CAD build for the part. Positions are in the model's coordinates, mm. A direction names the side the tool comes from. Give positions to 0.01 mm unless a question says otherwise; leave off trailing zeros. Loops run counter-clockwise (first coordinate to the right, second up) from the corner with the lowest first, then second, coordinate; pieces in that order, holes last. Notation, with made-up numbers: (-36, -1.5) -> (-29, -1.5) arc R9 cw to (-29, 7.5) -> close; hole circle Ø8 at (39, 70.25). An arc over 180 degrees is marked (long way). Write each question's results on one line, items separated by ' | '. Start each with the question number.
```python
from build123d import *

# Parameters (mm, degrees)
SKETCH_1_R          = 42
EXTRUDE_1_DEPTH     = 20
EXTRUDE_2_DEPTH     = 5
SKETCH_4_R          = 42
CUT_EXTRUDE_1_DEPTH = 15
SKETCH_5_R          = 42
EXTRUDE_3_DEPTH     = 10


with BuildPart() as part:
    # Sketch 1 → Extrude 1 (new body)
    with BuildSketch(Plane.XY):
        Circle(SKETCH_1_R)
    extrude(amount=EXTRUDE_1_DEPTH)



with BuildPart() as body_2:
    # Sketch 2 → Revolve 1 (revolve)
    with BuildSketch(Plane.XY.offset(20), mode=Mode.PRIVATE) as revolve_1_sk:
        with BuildLine():
            Line((100, 20), (100, 15))
            ThreePointArc((100, 15), (86.583592135, 6.708203932), (88, -9))
            Line((88, -9), (80, -9))
            Line((80, -9), (80, 20))
            Line((80, 20), (100, 20))
        make_face()
    revolve(revolve_1_sk.sketch.rotate(Axis((100, 22.717290725, 20), (0, -1, 0)), 270), axis=Axis((100, 22.717290725, 20), (0, -1, 0)))


with BuildPart() as part_1:
    add(part.part)

    add(body_2.part)  # Extrude 2 merges body 2
    # Sketch 3 → Extrude 2 (add, symmetric)
    with BuildSketch(Plane.XY.offset(20)):
        with BuildLine():
            Line((14.069453744, 39.573355574), (86, 14))
            Line((86, 14), (86, -3))
            Line((86, -3), (19.208719722, -37.350034627))
            ThreePointArc((19.208719722, -37.350034627), (-41.906577017, -2.79978619), (14.069453744, 39.573355574))
        make_face()
    extrude(amount=EXTRUDE_2_DEPTH, both=True)

    # Sketch 4 → Cut-Extrude 1 (cut)
    with BuildSketch(Plane(origin=(0, 0, 0), x_dir=(-1, 0, 0), z_dir=(0, 0, -1))):
        Circle(SKETCH_4_R)
    extrude(amount=-CUT_EXTRUDE_1_DEPTH, mode=Mode.SUBTRACT)

    # Sketch 5 → Extrude 3 (add)
    with BuildSketch(Plane.XY.offset(25)):
        with Locations(Location((0, 0, 0), (0, 0, 70.428252948))):
            Circle(SKETCH_5_R)
    extrude(amount=EXTRUDE_3_DEPTH)


solid = part_1.part
```
Q1. Mould opens along X. For faces 1 (the face through (55, 4, 25)), 2 (the face through (109, -9, 11)), 3 (the face through (119.524, 5.703, 15.664)) say: pulls with the +X half, pulls with the -X half, needs draft (parallel to the pull), parting line crosses it, or undercut.
Q2. Drop flat-ended pins along their axis: pin 1 (4 mm diameter, centred on y = -10, z = 16.5, fed in from +X); pin 2 (10 mm diameter, centred on x = 12, z = 32.5, fed in from +Y); pin 3 (8 mm diameter, centred on y = -16.5, z = 35, fed in from -X). Give the stop position or say it passes through.
Q3. Saw through at A-A, the plane y = 0. List the corners of the cut face in (x, z).
Q4. Saw through at B-B, the plane x = 0. List the corners of the cut face in (y, z), then the cut area to 3 significant figures.
Q5. Saw through at C-C, the plane y = 11. List the corners of the cut face in (x, z).
Q6. Saw through at D-D, the plane y = 36.5. List the corners of the cut face in (x, z), then the cut area to 3 significant figures.
Q7. Wall check: L1, parallel to Z at x = -18, y = 30.5; L2, parallel to Z at x = 69, y = 19.5; L3, parallel to Y at x = 88, z = 13.5. Give the ranges that are in metal, low to high.
Q8. Which spindle directions (+Z, -Z, +X, -X, +Y, -Y) get a long thin tool onto all of the face, cutting with end or side? Do faces 4 (the face through (-1, 0, 35)), 5 (the face through (100, 20, 20)), 6 (the face through (86, 1, 20)). Say none if no direction does.
Answer block:
1) face 1: undercut | face 2: needs draft | face 3: undercut
2) pin 1: stops at x = 119.92 | pin 2: stops at y = 41.41 | pin 3: stops at x = -40.1
3) outline: (-42, 15) -> (80.64, 15) arc R20 ccw (long way) to (80.64, 25) -> (42, 25) -> (42, 35) -> (-42, 35) -> close; hole (85.86, 15) arc R15 ccw (long way) to (85.86, 25) -> (86, 25) -> (86, 15) -> close
4) outline: (-42, 15) -> (42, 15) -> (42, 35) -> (-42, 35) -> close | area: 1,680 mm2
5) outline: (-40.53, 15) -> (80.64, 15) arc R20 ccw (long way) to (80.64, 25) -> (40.53, 25) -> (40.53, 35) -> (-40.53, 35) -> close; hole circle Ø20.4 at (100, 20)
6) outline: (-20.78, 15) -> (22.71, 15) -> (22.71, 25) -> (20.78, 25) -> (20.78, 35) -> (-20.78, 35) -> close | area: 850 mm2
7) L1: z = 15 to 35 | L2: z = 15 to 25 | L3: y = -9 to -6.22, 6.22 to 20
8) face 4: +Z, -X, +Y, -Y | face 5: +Z, -Z, +X, +Y | face 6: none
